from build123d import *

# Parameters (mm, degrees)
F1_DEPTH  = 127
F2_W      = 50.8
F2_H      = 704.724253
F3_DEPTH  = 127
F4_W      = 50.8
F4_H      = 711.2
F5_DEPTH  = 127
F6_W      = 495.3
F6_H      = 227.711381
F7_DEPTH  = 127
F8_W      = 38.1
F8_H      = 31.75
F9_DEPTH  = 495.3
F10_W     = 38.1
F10_H     = 39.75013
F11_DEPTH = 736.6
F12_W     = 38.1
F12_H     = 37.97719
F13_DEPTH = 736.6


with BuildPart() as f1:
    # F0 (on Front) → F1 (new body)
    with BuildSketch(Plane.XZ):
        Polygon((-227.385405, 388.756426), (-354.385405, 388.756426), (-354.385405, -385.943574), (394.914595, -385.943574), (394.914595, 388.756426), (267.914595, 388.756426), (267.914595, 1.406426), (-227.385405, 1.406426), align=None)
    extrude(amount=F1_DEPTH)

    # F2 (on face) → F3 (cut)
    with BuildSketch(Plane.XZ.offset(127)):
        with Locations((-290.885405, 4.644299)):
            Rectangle(F2_W, F2_H)
    extrude(amount=-F3_DEPTH, mode=Mode.SUBTRACT)

    # F4 (on face) → F5 (cut)
    with BuildSketch(Plane.XZ.offset(127)):
        with Locations((331.414595, 1.406426)):
            Rectangle(F4_W, F4_H)
    extrude(amount=-F5_DEPTH, mode=Mode.SUBTRACT)

    # F6 (on face) → F7 (cut)
    with BuildSketch(Plane.XZ.offset(127)):
        with Locations((20.264595, -233.987884)):
            Rectangle(F6_W, F6_H)
    extrude(amount=-F7_DEPTH, mode=Mode.SUBTRACT)

    # F8 (on face) → F9 (join)
    with BuildSketch(Plane.XZ.offset(127)):
        with Locations((-246.435405, 372.881426)):
            Rectangle(F8_W, F8_H)
        with Locations((286.964595, 372.881426)):
            Rectangle(F8_W, F8_H)
        with Locations((286.964595, -370.068574)):
            Rectangle(F8_W, F8_H)
        Polygon((-227.385405, -347.717827), (-265.485405, -347.717827), (-265.485405, -385.943574), (-227.385405, -385.943574), (-227.385405, -347.843574), align=None)
    extrude(amount=F9_DEPTH)

    # F10 (on face) → F11 (join)
    with BuildSketch(Plane(origin=(0, 0, 357.006426), x_dir=(1, 0, 0), z_dir=(0, 0, -1))):
        with Locations((-246.435405, 602.424935)):
            Rectangle(F10_W, F10_H)
    extrude(amount=F11_DEPTH)

    # F12 (on face) → F13 (join)
    with BuildSketch(Plane(origin=(0, 0, 357.006426), x_dir=(1, 0, 0), z_dir=(0, 0, -1))):
        with Locations((286.964595, 603.311405)):
            Rectangle(F12_W, F12_H)
    extrude(amount=F13_DEPTH)


solid = f1.part
Source: CAD feature listing. Evaluate the final solid. Frame: model axes, mm. A direction names the side the tool comes from. Coordinates: 2 decimals unless noted, no trailing zeros. Loops run counter-clockwise (first coordinate to the right, second up) from the corner with the lowest first, then second, coordinate; pieces in that order, holes last. Notation, with made-up numbers: (85.25, 43) -> (98.25, 43) arc R31 cw to (98.25, 78) -> close; hole circle Ø5 at (80, 9.5). An arc over 180 degrees is marked (long way). Answer in a Markdown table with one row per item. Add a question column.
Q1. Section D-D on y = -325.5. Return the cut outline in (x, z), and give its area (3 significant figures).
Q2. Pull-direction query (X, two-part tool) for faces 5 (the face through (287, -622.3, 7)), 6 (the face through (-291, -64, -347.718)), 7 (the face through (394.915, -63, -4)); classes: pulls with the +X half, pulls with the -X half, needs draft (parallel to the pull), parting line crosses it, or undercut.
Q3. Ray query, line 1 along X through (y, z) = (-81, 301); line 2 along Z through (x, y) = (-102, -65.5); line 3 along Y through (x, z) = (305.5, 312.5). Return the intervals inside material, ascending.
Q4. Section C-C on z = -323.5. Return the cut outline in (x, y).
Q5. Section A-A on x = 88. Return the cut outline in (y, z).
Q6. Section B-B on y = -76.5. Return the cut outline in (x, z).
Q7. Reachability of faces 1 (the face through (-264, -238, 388.756)), 2 (the face through (-265.485, -125, 32)), 3 (the face through (17, -64, -120.132)), 4 (the face through (-246, -352, -347.718)) from +Z, -Z, +X, -X, +Y, -Y: full face, straight path, thin tool, end or side. Return the list, or none.
Computed values:
| question | item | result |
|---|---|---|
| 1 | outline | (-265.49, -385.94) -> (-227.39, -385.94) -> (-227.39, -347.72) -> (-265.49, -347.72) -> close; (-265.49, 357.01) -> (-227.39, 357.01) -> (-227.39, 388.76) -> (-265.49, 388.76) -> close; (267.91, -385.94) -> (306.01, -385.94) -> (306.01, -354.19) -> (267.91, -354.19) -> close; (267.91, 357.01) -> (306.01, 357.01) -> (306.01, 388.76) -> (267.91, 388.76) -> close |
| 1 | area | 5,090 mm^2 |
| 2 | face 5 | needs draft |
| 2 | face 6 | undercut |
| 2 | face 7 | pulls with the +X half |
| 3 | line 1 | x = -354.39 to -316.29, -265.49 to -227.39, 267.91 to 306.01, 356.81 to 394.91 |
| 3 | line 2 | z = -385.94 to -347.84, -120.13 to 1.41 |
| 3 | line 3 | y = -622.3 to -584.32, -127 to 0 |
| 4 | outline | (-354.39, -127) -> (-316.29, -127) -> (-316.29, 0) -> (-354.39, 0) -> close; (-265.49, -622.3) -> (-227.39, -622.3) -> (-227.39, -582.55) -> (-265.49, -582.55) -> close; (-265.49, -127) -> (-227.39, -127) -> (-227.39, 0) -> (-265.49, 0) -> close; (267.91, -622.3) -> (306.01, -622.3) -> (306.01, -584.32) -> (267.91, -584.32) -> close; (267.91, -127) -> (306.01, -127) -> (306.01, 0) -> (267.91, 0) -> close; (356.81, -127) -> (394.91, -127) -> (394.91, 0) -> (356.81, 0) -> close |
| 5 | outline | (-127, -385.94) -> (0, -385.94) -> (0, -347.84) -> (-127, -347.84) -> close; (-127, -120.13) -> (0, -120.13) -> (0, 1.41) -> (-127, 1.41) -> close |
| 6 | outline | (-354.39, -385.94) -> (394.91, -385.94) -> (394.91, 388.76) -> (267.91, 388.76) -> (267.91, 1.41) -> (-227.39, 1.41) -> (-227.39, 388.76) -> (-354.39, 388.76) -> close; hole (-316.29, -347.72) -> (-265.49, -347.72) -> (-265.49, 357.01) -> (-316.29, 357.01) -> close; hole (-227.39, -347.84) -> (267.91, -347.84) -> (267.91, -120.13) -> (-227.39, -120.13) -> close; hole (306.01, -354.19) -> (356.81, -354.19) -> (356.81, 357.01) -> (306.01, 357.01) -> close |
| 7 | face 1 | +Z, +X, -X, +Y, -Y |
| 7 | face 2 | +Y, -Y |
| 7 | face 3 | +Y, -Y |
| 7 | face 4 | +X, -X |
